Could you check a few things on this model? Use its own coordinates, in mm. Face numbers are marked on the shaded views. A direction names the side the tool comes from. Round coordinates to 2 decimals unless told otherwise and drop trailing zeros. Order: outer loops, then holes, each group sorted by start corner. A loop starts at its lowest first (then second) coordinate and runs counter-clockwise, first axis right, second up.
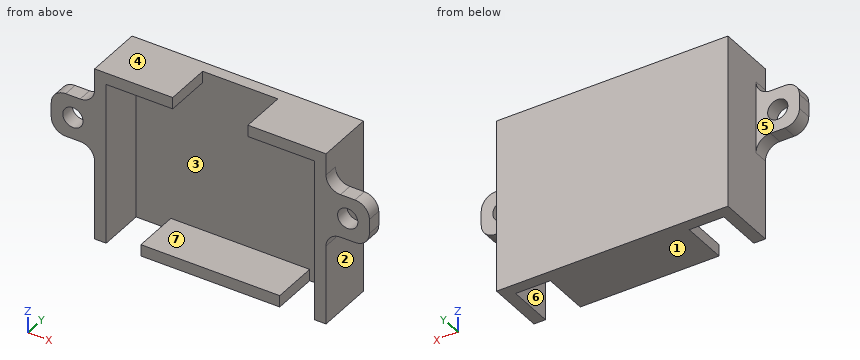
```python
from build123d import *

# Parameters (mm, degrees)
SKETCH1_W           = 40
SKETCH1_H           = 30
BOSS_EXTRUDE1_DEPTH = 10
CUT_EXTRUDE1_DEPTH  = 8
SKETCH3_W           = 7.5
SKETCH3_H           = 2.5
BOSS_EXTRUDE2_DEPTH = 7.5
SKETCH4_R           = 1.75
CUT_EXTRUDE2_DEPTH  = 51.55937104
FILLET1_R           = 2.5
FILLET2_R           = 2.5


with BuildPart() as part:
    # Sketch1 → Boss-Extrude1 (new body)
    with BuildSketch(Plane(origin=(0, 0, 0), x_dir=(1, 0, 0), z_dir=(0, 1, 0))):
        with Locations((20, 15)):
            Rectangle(SKETCH1_W, SKETCH1_H)
    extrude(amount=BOSS_EXTRUDE1_DEPTH)

    # Sketch2 → Cut-Extrude1 (cut)
    with BuildSketch(Plane.XZ):
        Polygon((13.5, 0), (26.5, 0), (26.5, -2), (38, -2), (38, -28), (38, -30), (32, -30), (32, -28), (8, -28), (8, -30), (2, -30), (2, -28), (2, -2), (13.5, -2), align=None)
    extrude(amount=-CUT_EXTRUDE1_DEPTH, mode=Mode.SUBTRACT)

    # Sketch3 → Boss-Extrude2 (add)
    with BuildSketch(Plane.ZY):
        with Locations((-10, 1.25)):
            Rectangle(SKETCH3_W, SKETCH3_H)
    boss_extrude2 = extrude(amount=BOSS_EXTRUDE2_DEPTH)

    # Sketch4 → Cut-Extrude2 (cut, through all)
    with BuildSketch(Plane(origin=(0, 2.5, 0), x_dir=(1, 0, 0), z_dir=(0, 1, 0))):
        with Locations(Location((-3.75, 10, 0), (0, 0, 270))):
            Circle(SKETCH4_R)
    cut_extrude2 = extrude(amount=-CUT_EXTRUDE2_DEPTH, mode=Mode.SUBTRACT)

    # Fillet1
    fillet1_edges = [part.edges().sort_by_distance(p)[0] for p in [
        (0, 1.25, -6.25),
        (0, 1.25, -13.75),
        (-7.5, 1.25, -6.25),
        (-7.5, 1.25, -13.75),
    ]]
    fillet(fillet1_edges, radius=FILLET1_R)

    # Mirror1: Boss-Extrude2, Cut-Extrude2 across plane
    add(boss_extrude2.mirror(Plane.ZY.offset(-20)))
    add(cut_extrude2.mirror(Plane.ZY.offset(-20)), mode=Mode.SUBTRACT)

    # Fillet2
    fillet2_edges = [part.edges().sort_by_distance(p)[0] for p in [
        (47.5, 1.25, -6.25),
        (47.5, 1.25, -13.75),
        (40, 1.25, -6.25),
        (40, 1.25, -13.75),
    ]]
    fillet(fillet2_edges, radius=FILLET2_R)


solid = part.part
```
Q1. Imagine slicing it at C-C, the plane x = 43.75. Please give me the cut outline in (y, z).
Q2. I need wall thicknesses on L1, parallel to X at y = 0.65, z = -10; L2, parallel to X at y = 3.5, z = -4; L3, parallel to Z at x = 43.75, y = 0.95. Which ranges of each line are inside material? Lowest first, please.
Q3. We'd pull the mould along Z, two halves only. Please class the marked faces 1, 2, 3 and 4: released by +Z, released by -Z, zero draft, split by the parting line, or undercut.
Q4. Imagine slicing it at D-D, the plane x = 22.5. Please give me the cut outline in (y, z), then the cut area to 3 significant figures.
Q5. Imagine slicing it at B-B, the plane z = -10. Please give me the cut outline in (x, y).
Q6. For P1, Ø1.5, axis at x = 26.5, y = 2.5, coming from the +Z side; P2, Ø2, axis at y = 4, z = -1, coming from the +X side; P3, Ø2, axis at x = 43.5, y = 1, coming from the -Z side; P4, Ø3, axis at y = 7, z = -9, coming from the -X side, each with a flat end and sliding along its axis, tell me the tip position at first contact or that it passes through.
Q7. For the marked faces 5, 6 and 7, which set-ups out of +Z, -Z, +X, -X, +Y, -Y let a thin tool reach every point of the face, with its end or its side?
Q8. Imagine slicing it at A-A, the plane y = 5.25. Please give me the cut outline in (x, z), then the cut area to 3 significant figures.
Filled in:
1. outline: (0, -13.75) - (2.5, -13.75) - (2.5, -11.75) - (0, -11.75) - close; (0, -8.25) - (2.5, -8.25) - (2.5, -6.25) - (0, -6.25) - close
2. L1: x = -7.5 to -5.5, -2 to 2, 38 to 42, 45.5 to 47.5
2. L2: x = 0 to 2, 38 to 40
2. L3: z = -13.75 to -11.75, -8.25 to -6.25
3. face 1: released by -Z
3. face 2: zero draft
3. face 3: undercut
3. face 4: released by +Z
4. outline: (0, -30) - (10, -30) - (10, 0) - (8, 0) - (8, -28) - (0, -28) - close
4. area: 76.0 mm2
5. outline: (-7.5, 0) - (-5.5, 0) - (-5.5, 2.5) - (-7.5, 2.5) - close; (-2, 0) - (2, 0) - (2, 8) - (38, 8) - (38, 0) - (42, 0) - (42, 2.5) - (40, 2.5) - (40, 10) - (0, 10) - (0, 2.5) - (-2, 2.5) - close; (45.5, 0) - (47.5, 0) - (47.5, 2.5) - (45.5, 2.5) - close
6. P1: stops at z = 0
6. P2: stops at x = 40
6. P3: stops at z = -13.75
6. P4: stops at x = 0
7. face 5: +Z, -Z, -X, +Y
7. face 6: -Z, -Y
7. face 7: -Y
8. outline: (0, -30) - (2, -30) - (2, -2) - (13.5, -2) - (13.5, 0) - (0, 0) - close; (8, -30) - (32, -30) - (32, -28) - (8, -28) - close; (26.5, -2) - (38, -2) - (38, -30) - (40, -30) - (40, 0) - (26.5, 0) - close
8. area: 214 mm2
